```python
from build123d import *

# Parameters (mm, degrees)
F1_DEPTH = 36
F3_DEPTH = 5
F5_DEPTH = 5
F6_DEPTH = 22
F7_DEPTH = 14


with BuildPart() as f1:
    # F0 (on Right) → F1 (new body)
    with BuildSketch(Plane.YZ):
        Polygon((-64.146131, 8), (-64.146131, 0), (-43.146131, 0), (-32.146131, 32), (-4.146131, 32), (6.853869, 0), (27.853869, 0), (27.853869, 8), (12.563331, 8), (0.937467, 41.820695), (-28.062533, 41.820695), (-37.689707, 41.820695), (-48.855593, 8), align=None)
    extrude(amount=F1_DEPTH)

    # F2 (on face) → F3 (cut)
    with BuildSketch(Plane.YZ.offset(36)):
        Polygon((-37.689707, 41.820695), (-48.855593, 8), (-40.396131, 8), (-32.146131, 32), (-4.146131, 32), (4.103869, 8), (12.563331, 8), (0.937467, 41.820695), align=None)
    extrude(amount=-F3_DEPTH, mode=Mode.SUBTRACT)

    # F4 (on face) → F5 (cut)
    with BuildSketch(Plane(origin=(0, 0, 0), x_dir=(0, -1, 0), z_dir=(-1, 0, 0))):
        Polygon((-0.937467, 41.820695), (-12.563331, 8), (-4.103869, 8), (4.146131, 32), (32.146131, 32), (40.396131, 8), (48.855593, 8), (37.689707, 41.820695), align=None)
    extrude(amount=-F5_DEPTH, mode=Mode.SUBTRACT)

    # F0 (on Right) → F6 (join)
    with BuildSketch(Plane.YZ):
        Polygon((-37.689707, 41.820695), (-64.146131, 8), (-48.855593, 8), align=None)
    extrude(amount=F6_DEPTH)

    # F0 (on Right) → F7 (cut)
    with BuildSketch(Plane.YZ):
        Polygon((-37.689707, 41.820695), (-64.146131, 8), (-48.855593, 8), align=None)
    extrude(amount=F7_DEPTH, mode=Mode.SUBTRACT)


solid = f1.part
```
For this review, take the finished solid that the model builds, in its own axes (mm). A direction names the side the tool comes from. Round coordinates to 2 decimals unless told otherwise and drop trailing zeros. Write each loop counter-clockwise with the first axis right and the second up, starting at its lowest first coordinate (ties: lowest second). Pieces come first, ordered by that corner, then holes. Notation, with made-up numbers: (52, 67.5) - (87, 67.5) arc R16 ccw to (87, 93.5) - close; hole circle Ø5 at (85.5, 88). An arc over 180 degrees is marked (long way). Put each result on its own line as item: value.
Q1. Machinability: for faces 1 (the face through (31, -19, 33)), 2 (the face through (29, -55, 8)), 3 (the face through (5, -18, 33)), 4 (the face through (7, -55, 8)), which of the approach directions +Z, -Z, +X, -X, +Y, -Y give a long, thin tool a straight path to every point of the face, cutting with its end or side? Answer none if there is none.
Solved:
face 1: +Z, +X, +Y, -Y
face 2: +Z, +X, -Y
face 3: +Z, -X, +Y, -Y
face 4: +Z, -X, -Y
Q2. We need section B-B (z = 10). Give the boundary of the cut face in (x, y).
Solved:
outline: (5, -48.2) - (14, -48.2) - (14, -62.58) - (22, -62.58) - (22, -48.2) - (31, -48.2) - (31, -39.71) - (5, -39.71) - close; (5, 3.42) - (31, 3.42) - (31, 11.88) - (5, 11.88) - close
Q3. Mouldability with a two-part tool opening along Y and no side actions: class faces 5 (the face through (9.44, -43.35, 24.67)), 6 (the face through (17.818, 6.832, 24.674)), 7 (the face through (17.75, -37.72, 15.78)), 8 (the face through (22, -50, 20)) as released by +Y, released by -Y, zero draft, split by the parting line, or undercut.
Solved:
face 5: released by -Y
face 6: released by +Y
face 7: undercut
face 8: zero draft
Q4. Wall thickness on probe 1 along Z at (x, y) = (17.5, 16.5); probe 2 along X at (y, z) = (-33, 30); probe 3 along Z at (x, y) = (7, -16): over which ranges is each line inside the solid? List them lowest first.
Solved:
probe 1: z = 0 to 8
probe 2: x = 5 to 31
probe 3: z = 32 to 41.82
Q5. Insertion check: pin 1 Ø3 at (x, z) = (24.5, 20) entering from -Y; pin 2 Ø6 at (x, z) = (22.5, 26.5) entering from +Y; pin 3 Ø8 at (y, z) = (-45.5, 18.5) entering from -X; pin 4 Ø1 at (x, y) = (32, -54) entering from -Z. Each pin has a flat end and moves straight along its axis. Give the tip position at first contact, or say it passes through.
Solved:
pin 1: stops at y = -45.39
pin 2: stops at y = 7.24
pin 3: stops at x = 5
pin 4: stops at z = 0
Q6. We need section C-C (x = 13). Give the boundary of the cut face in (y, z).
Solved:
outline: (-64.15, 0) - (-43.15, 0) - (-32.15, 32) - (-4.15, 32) - (6.85, 0) - (27.85, 0) - (27.85, 8) - (12.56, 8) - (0.94, 41.82) - (-37.69, 41.82) - (-48.86, 8) - (-64.15, 8) - close
Q7. We need section D-D (y = -46). Give the boundary of the cut face in (x, z), and give its area (3 significant figures).
Solved:
outline: (0, 0) - (36, 0) - (36, 8) - (31, 8) - (31, 16.65) - (22, 16.65) - (22, 31.2) - (14, 31.2) - (14, 16.65) - (5, 16.65) - (5, 8) - (0, 8) - close
area: 629 mm2
Q8. We need section A-A (x = 3). Give the boundary of the cut face in (y, z), and give its area (3 significant figures).
Solved:
outline: (-64.15, 0) - (-43.15, 0) - (-40.4, 8) - (-64.15, 8) - close; (4.1, 8) - (6.85, 0) - (27.85, 0) - (27.85, 8) - close
area: 358 mm2
